Could you check a few things on this model? Use its own coordinates, in mm. A direction names the side the tool comes from. Coordinates: 2 decimals unless noted, no trailing zeros. Loops run counter-clockwise (first coordinate to the right, second up) from the corner with the lowest first, then second, coordinate; pieces in that order, holes last. Notation, with made-up numbers: (26, 56.25) -> (51, 56.25) arc R23 ccw to (51, 79.25) -> close; hole circle Ø10 at (72, -34). An arc over 180 degrees is marked (long way). One line per question, with ' | ' between items. Start each with the question number.
(1) I'm going to push flat-ended pins straight in: pin 1 Ø1.5 at (x, y) = (-12, 9.5) entering from -Z; pin 2 Ø2 at (x, y) = (-14, -1) entering from +Z; pin 3 Ø5.5 at (x, z) = (-4, 11) entering from +Y; pin 4 Ø5.5 at (y, z) = (-5.5, 2) entering from -X. Where does each tip first touch, or does it pass through?
(2) Which directions (+Z, -Z, +X, -X, +Y, -Y) give clear straight access to the entire face, cutting with the end or side of a thin tool? Please do faces 5 (the face through (10.55, 7, 4)), 6 (the face through (-14.645, -13.081, 14.126)), 7 (the face through (-13.2, 8.6, 2.5)), 8 (the face through (15, -2, 1)), 9 (the face through (13, -6, 4)).
(3) Suppose I cut it at C-C (x = -18.5). Please give me the cut outline in (y, z), plus the area to 3 significant figures.
(4) If I drill on line 1 along Z through (x, y) = (19, -13.65); line 2 along Y through (x, z) = (-13, 4); line 3 along Y through (x, z) = (-12.85, 1), over which ranges is the centre line in solid material (lowest first)?
(5) Suppose I cut it at B-B (z = 3.5). Give the number of separate pieces and of enclosed holes in the cut face, plus the area to 3 significant figures.
(6) Suppose I cut it at D-D (x = -6). Please give me the cut outline in (y, z), plus the area to 3 significant figures.
(7) Suppose I cut it at A-A (z = 18.5). Please give me the cut outline in (x, y).
(8) If we mould it in two halves opening along Y, with no side actions, what happens to faces 1 (the face through (2, 0, 2)), 2 (the face through (13, 6, 4)), 3 (the face through (-15, -2, 2)), 4 (the face through (0, -13.3, 14))? For each: pulls with the +Y half, pulls with the -Y half, needs draft (parallel to the pull), parting line crosses it, or undercut.
```python
from build123d import *

# Parameters (mm, degrees)
SKETCH_1_W          = 30
SKETCH_1_H          = 25
EXTRUDE_1_DEPTH     = 5
SKETCH_2_W          = 21.1
SKETCH_2_H          = 15.1
CUT_EXTRUDE_1_DEPTH = 3
SKETCH_3_W          = 4.45
SKETCH_3_H          = 12
CUT_EXTRUDE_2_DEPTH = 3
FILLET_3_R          = 3
SKETCH_8_R          = 1.5
CUT_EXTRUDE_6_DEPTH = 10
SKETCH_9_W          = 47
SKETCH_9_H          = 23
EXTRUDE_2_DEPTH     = 3
SKETCH_10_R         = 1.5
CUT_EXTRUDE_7_DEPTH = 42.306779105
FILLET_4_R          = 2
SKETCH_11_W         = 30
SKETCH_11_H         = 0.8
CUT_EXTRUDE_8_DEPTH = 18
FILLET_5_R          = 1


with BuildPart() as part:
    # 草图1 → 凸台-拉伸1 (new body)
    with BuildSketch(Plane.XY):
        Rectangle(SKETCH_1_W, SKETCH_1_H)
    extrude(amount=EXTRUDE_1_DEPTH)

    # 草图2 → 切除-拉伸1 (cut)
    with BuildSketch(Plane.XY.offset(5)):
        Rectangle(SKETCH_2_W, SKETCH_2_H)
    extrude(amount=-CUT_EXTRUDE_1_DEPTH, mode=Mode.SUBTRACT)

    # 草图3 → 切除-拉伸2 (cut)
    with BuildSketch(Plane.XY.offset(5)):
        with Locations((12.775, 0)):
            Rectangle(SKETCH_3_W, SKETCH_3_H)
    extrude(amount=-CUT_EXTRUDE_2_DEPTH, mode=Mode.SUBTRACT)

    # 圆角3
    fillet_3_edges = [part.edges().sort_by_distance(p)[0] for p in [
        (-15, 12.5, 2.5),
        (15, 12.5, 2.5),
    ]]
    fillet(fillet_3_edges, radius=FILLET_3_R)

    # 草图8 → 切除-拉伸6 (cut, symmetric)
    with BuildSketch(Plane.XY.offset(2)):
        with Locations((12, 9.5)):
            Circle(SKETCH_8_R)
        with Locations((-12, 9.5)):
            Circle(SKETCH_8_R)
        with Locations((-12.85, -0.55)):
            Circle(SKETCH_8_R)
    extrude(amount=CUT_EXTRUDE_6_DEPTH, both=True, mode=Mode.SUBTRACT)

    # 草图9 → 凸台-拉伸2 (add)
    with BuildSketch(Plane.XZ.offset(12.5)):
        with Locations((0, 11.5)):
            Rectangle(SKETCH_9_W, SKETCH_9_H)
    extrude(amount=EXTRUDE_2_DEPTH)

    # 草图10 → 切除-拉伸7 (cut, through all)
    with BuildSketch(Plane(origin=(0, -12.5, 0), x_dir=(1, 0, 0), z_dir=(0, 1, 0))):
        with Locations(Location((-19, -3.5, 0), (0, 0, 180))):
            Circle(SKETCH_10_R)
        with Locations(Location((19, -3.5, 0), (0, 0, 180))):
            Circle(SKETCH_10_R)
        with Locations(Location((-19, -18.5, 0), (0, 0, 180))):
            Circle(SKETCH_10_R)
        with Locations(Location((19, -18.5, 0), (0, 0, 180))):
            Circle(SKETCH_10_R)
    extrude(amount=-CUT_EXTRUDE_7_DEPTH, mode=Mode.SUBTRACT)

    # 圆角4
    fillet_4_edges = [part.edges().sort_by_distance(p)[0] for p in [
        (-23.5, -14, 23),
        (-23.5, -14, 0),
        (23.5, -14, 0),
        (23.5, -14, 23),
    ]]
    fillet(fillet_4_edges, radius=FILLET_4_R)

    # 草图11 → 切除-拉伸8 (cut)
    with BuildSketch(Plane.XY.offset(23)):
        with Locations((0, -12.9)):
            Rectangle(SKETCH_11_W, SKETCH_11_H)
    extrude(amount=-CUT_EXTRUDE_8_DEPTH, mode=Mode.SUBTRACT)

    # 圆角5
    # the kernel refuses this fillet: 1 mm, written as the material it adds along each edge
    with BuildSketch(Plane(origin=(15, -13.3, 23), x_dir=(-1.569855356819468e-12, 1.0, 0), z_dir=(0, 0, -1))) as fillet_5_piece_1:
        with BuildLine():
            CenterArc((1, -0.979795897), FILLET_5_R, 101.536959033, 78.463040967)
            Line((0, -0.979795897), (-0.02, -0.979795897))
            Line((-0.02, -0.979795897), (-0.02, 0))
            Line((-0.02, 0), (0, 0.02))
            ThreePointArc((0, 0.02), (0.4, 0.02), (0.796, 0.019595918))
            Line((0.796, 0.019595918), (0.8, 0))
        make_face()
    extrude(amount=20.449489743)
    with BuildSketch(Plane(origin=(-15, -13.3, 23), x_dir=(1.5720758028687176e-12, 1.0, 0), z_dir=(0, 0, -1))) as fillet_5_piece_2:
        with BuildLine():
            CenterArc((1, 0.979795897), FILLET_5_R, 180, 78.463040967)
            Line((0, 0.979795897), (-0.02, 0.979795897))
            Line((-0.02, 0.979795897), (-0.02, 0))
            Line((-0.02, 0), (0, -0.02))
            ThreePointArc((0, -0.02), (0.4, -0.02), (0.796, -0.019595918))
            Line((0.796, -0.019595918), (0.8, 0))
        make_face()
    extrude(amount=20.449489743)


solid = part.part
```
Checks:
1) pin 1: passes through | pin 2: stops at z = 5 | pin 3: stops at y = -13.3 | pin 4: stops at x = -15
2) face 5: +Z | face 6: +Z, +Y | face 7: +Z, -Z | face 8: +Z, -Z, +X, +Y | face 9: +Z, +X
3) outline: (-15.5, 0) -> (-12.5, 0) -> (-12.5, 2.09) -> (-15.5, 2.09) -> close; (-15.5, 4.91) -> (-12.5, 4.91) -> (-12.5, 17.09) -> (-15.5, 17.09) -> close; (-15.5, 19.91) -> (-12.5, 19.91) -> (-12.5, 23) -> (-15.5, 23) -> close | area: 52.0 mm^2
4) line 1: z = 0 to 2, 5 to 17, 20 to 23 | line 2: y = -15.5 to -2.04, 0.94 to 8.38, 10.62 to 12.33 | line 3: y = -15.5 to -2.05, 0.95 to 8.26, 10.74 to 12.38
5) separate pieces: 3 | enclosed holes: 3 | area: 476 mm^2
6) outline: (-15.5, 0) -> (12.5, 0) -> (12.5, 5) -> (7.55, 5) -> (7.55, 2) -> (-7.55, 2) -> (-7.55, 5) -> (-13.3, 5) -> (-13.3, 23) -> (-15.5, 23) -> close | area: 134 mm^2
7) outline: (-23.5, -15.5) -> (-20.5, -15.5) -> (-20.5, -12.5) -> (-23.5, -12.5) -> close; (-17.5, -15.5) -> (17.5, -15.5) -> (17.5, -12.5) -> (15, -12.5) arc R1 cw to (14.02, -13.3) -> (-14.02, -13.3) arc R1 cw to (-15, -12.5) -> (-17.5, -12.5) -> close; (20.5, -15.5) -> (23.5, -15.5) -> (23.5, -12.5) -> (20.5, -12.5) -> close
8) face 1: undercut | face 2: undercut | face 3: needs draft | face 4: pulls with the +Y half
